from build123d import *

# Parameters (mm, degrees)
SKETCH1_R           = 1.45
SKETCH1_R_2         = 1.5
BOSS_EXTRUDE1_DEPTH = 1.5
FILLET1_R           = 10


with BuildPart() as part:
    # Sketch1 → Boss-Extrude1 (new, symmetric)
    with BuildSketch(Plane(origin=(0, 0, 0), x_dir=(0, 0, -1), z_dir=(1, 0, 0))):
        with BuildLine():
            Line((-110, 14), (-127.759109434, 6.974045822))
            ThreePointArc((-127.759109434, 6.974045822), (-132.233383985, -1.981957648), (-123.818844483, -7.406407472))
            Line((-123.818844483, -7.406407472), (-115, -6))
            Line((-115, -6), (-91, -4.5))
            Line((-91, -4.5), (-6, -4.5))
            ThreePointArc((-6, -4.5), (0, -7.5), (6, -4.5))
            Line((6, -4.5), (39.334317565, -7.47039938))
            ThreePointArc((39.334317565, -7.47039938), (47.425031601, -1.057783404), (41.446954522, 7.359097948))
            Line((41.446954522, 7.359097948), (-2.5, 16))
            Line((-2.5, 16), (-110, 14))
        make_face()
        with Locations((-125, 0)):
            Circle(SKETCH1_R, mode=Mode.SUBTRACT)
        Circle(SKETCH1_R, mode=Mode.SUBTRACT)
        with Locations((-106.5, 5)):
            Circle(SKETCH1_R_2, mode=Mode.SUBTRACT)
        Polygon((-33, 8.5), (-31.5, 7), (-31.5, 3), (-33, 1.5), (-97, 1.5), (-98.5, 3), (-98.5, 7), (-97, 8.5), align=None, mode=Mode.SUBTRACT)
        with Locations((-23.5, 8.5)):
            Circle(SKETCH1_R_2, mode=Mode.SUBTRACT)
        with Locations((40, 0)):
            Circle(SKETCH1_R, mode=Mode.SUBTRACT)
    extrude(amount=BOSS_EXTRUDE1_DEPTH, both=True)

    # Fillet1
    # the kernel refuses this fillet: 10 mm, written as the material it adds along each edge
    with BuildSketch(Plane(origin=(-1.5, -4.5, -6), x_dir=(0, -0.08875765800116116, -0.9960532506578896), z_dir=(1, 0, 0))) as fillet1_piece_1:
        with BuildLine():
            CenterArc((4.191013496, -10), FILLET1_R, 90, 37.143535998)
            ThreePointArc((-1.847125053, -2.028746469), (-0.83000341, -1.099556568), (0, 0))
            Line((0, 0), (4.191013496, 0))
        make_face()
    extrude(amount=3)
    with BuildSketch(Plane(origin=(-1.5, -4.5, 6), x_dir=(0, -0.689479455343069, -0.7243052399781633), z_dir=(1, 0, 0))) as fillet1_piece_2:
        with BuildLine():
            CenterArc((4.143912969, -9.861667083), FILLET1_R, 99.541184992, 34.04773237)
            Line((-2.750881584, -2.618614683), (0, 0))
            ThreePointArc((0, 0), (1.243173891, -0.103749688), (2.486347782, 0))
        make_face()
    extrude(amount=3)
    with BuildSketch(Plane(origin=(-1.5, -4.5, 91), x_dir=(0, 0, -1), z_dir=(1, 0, 0))) as fillet1_piece_3:
        with BuildLine():
            CenterArc((FILLET1_R * 0.0312195418814, -FILLET1_R), FILLET1_R, 90, 3.576334375)
            Line((-FILLET1_R * 0.0311587442738, -FILLET1_R * 0.00194742151711), (0, 0))
            Line((0, 0), (FILLET1_R * 0.0312195418814, 0))
        make_face()
    extrude(amount=3)
    with BuildSketch(Plane(origin=(-1.5, -6, 115), x_dir=(0, 0.06237828615518053, -0.9980525784828885), z_dir=(1, 0, 0))) as fillet1_piece_4:
        with BuildLine():
            CenterArc((FILLET1_R * 0.04790007143, -FILLET1_R), FILLET1_R, 90, 5.484751657)
            Line((-FILLET1_R * 0.0476807691396, -FILLET1_R * 0.00457832909063), (0, 0))
            Line((0, 0), (FILLET1_R * 0.04790007143, 0))
        make_face()
    extrude(amount=3)
    # the kernel refuses this fillet: 10 mm, written as the material it takes off along each edge
    with BuildSketch(Plane(origin=(-6.025054026, 14, 110), x_dir=(0, 0.018601432156142118, -0.9998269783926319), z_dir=(1, 0, 0))) as fillet1_2_piece_1:
        with BuildLine():
            CenterArc((FILLET1_R * 0.181002161022, -FILLET1_R), FILLET1_R, 90, 20.51916315)
            Line((-FILLET1_R * 0.169518480088, -FILLET1_R * 0.0634449935237), (0, 0))
            Line((0, 0), (FILLET1_R * 0.181002161022, 0))
        make_face()
    extrude(amount=12.050108051, mode=Mode.SUBTRACT)
    with BuildSketch(Plane(origin=(4.169414773, 16, 2.5), x_dir=(0, -0.018601432156142392, 0.9998269783926319), z_dir=(-1, 0, 0))) as fillet1_2_piece_2:
        with BuildLine():
            CenterArc((FILLET1_R * 0.106776590902, -FILLET1_R), FILLET1_R, 90, 12.189510847)
            Line((-FILLET1_R * 0.104369266233, -FILLET1_R * 0.0225454348081), (0, 0))
            Line((0, 0), (FILLET1_R * 0.106776590902, 0))
        make_face()
    extrude(amount=8.338829545, mode=Mode.SUBTRACT)


solid = part.part
Geometry: final body of the model. Coordinates: model frame, mm. A direction names the side the tool comes from. Coordinates: 2 decimals unless noted, no trailing zeros. Loops run counter-clockwise (first coordinate to the right, second up) from the corner with the lowest first, then second, coordinate; pieces in that order, holes last. Notation, with made-up numbers: (-3.5, 65.5) - (6.5, 65.5) arc R19 cw to (6.5, 92.5) - close; hole circle Ø5 at (-22.5, 65). An arc over 180 degrees is marked (long way). Put each result on its own line as item: value. Start each with the question number.
Q1. Cut plane B-B, the plane y = 5. Return loops of the section in (x, z).
Q2. Line query: line 1 (Z direction, x = -0.8, y = 3.75); line 2 (Y direction, x = 0.2, z = 107.5); line 3 (Z direction, x = 0.05, y = 0.75). Output: solid intervals per line, ascending.
Q3. Pin query (flat end, axial travel): pin 1 Ø2.5 at (y, z) = (5, 106.5) entering from -X; pin 2 Ø0.9 at (x, z) = (0, 66) entering from -Y; pin 3 Ø0.9 at (x, y) = (0.5, 4.5) entering from +Z. Return the tip coordinate at first contact, or that it passes through.
Q4. Cut plane C-C, the plane z = 106.5. Return loops of the section in (x, y), and give its area (3 significant figures).
Q5. Set-up query: faces 5 (the flat face through (-1.5, 0, 41)), 6 (the flat face through (0, 8.5, 65)), 7 (the flat face through (0.021, -6.153, -24.55)). Return all of +Z, -Z, +X, -X, +Y, -Y with unobstructed straight access to the full face (end or side cutting, diameter ignored); none if empty.
Q6. Cut plane D-D, the plane z = 23.5. Return loops of the section in (x, y).
Q7. Pull-direction query (Y, two-part tool) for faces 1 (the flat face through (1.5, 0, 41)), 2 (the flat face through (0, 1.5, 65)), 3 (the flat face through (0, 5, 98.5)), 4 (the flat face through (0.021, -5.255, 103.079)); classes: released by +Y, released by -Y, zero draft, split by the parting line, or undercut.
Q8. Cut plane A-A, the plane x = 0.65. Give the number of separate pieces and of enclosed holes in the cut face, and give its area (3 significant figures).
Filled sheet:
1. outline: (-1.5, -45.59) - (1.5, -45.59) - (1.5, 31.5) - (-1.5, 31.5) - close; (-1.5, 98.5) - (1.5, 98.5) - (1.5, 105) - (-1.5, 105) - close; (-1.5, 108) - (1.5, 108) - (1.5, 130.59) - (-1.5, 130.59) - close
2. line 1: -46.5 to 31.5, 98.5 to 105.67, 107.33 to 131.5
2. line 2: -5.53 to 3.88, 6.12 to 14.05
2. line 3: -47.46 to -41.24, -38.76 to -1.24, 1.24 to 123.76, 126.24 to 132.46
3. pin 1: through
3. pin 2: y = -4.5
3. pin 3: z = 131.31
4. outline: (-1.5, -5.47) - (1.5, -5.47) - (1.5, 3.5) - (-1.5, 3.5) - close; (-1.5, 6.5) - (1.5, 6.5) - (1.5, 14.07) - (-1.5, 14.07) - close
4. area: 49.6 mm²
5. face 5: +Z, -Z, -X, +Y, -Y
5. face 6: +X, -X
5. face 7: +X, -X, -Y
6. outline: (-1.5, -4.5) - (1.5, -4.5) - (1.5, 7) - (-1.5, 7) - close; (-1.5, 10) - (1.5, 10) - (1.5, 15.61) - (-1.5, 15.61) - close
7. face 1: zero draft
7. face 2: undercut
7. face 3: undercut
7. face 4: released by -Y
8. separate pieces: 1
8. enclosed holes: 6
8. area: 2,820 mm²
